The model under review builds one solid part; all positions refer to its coordinate system, in mm. Face numbers are marked on the shaded views. Round coordinates to 2 decimals unless told otherwise and drop trailing zeros. Loops run counter-clockwise (first coordinate to the right, second up) from the corner with the lowest first, then second, coordinate; pieces in that order, holes last. Notation, with made-up numbers: (-32, 39.5) -> (-9, 39.5) arc R5 cw to (-9, 48.5) -> close; hole circle Ø7 at (8, 71.25). An arc over 180 degrees is marked (long way). Return JSON: item names as keys, results as strings. Group by question number.
```python
from build123d import *

# Parameters (mm, degrees)
AUFSATZ_LINEAR_AUSTRAGEN1_DEPTH = 500


with BuildPart() as part:
    # Skizze1 → Aufsatz-Linear austragen1 (new body, symmetric)
    with BuildSketch(Plane(origin=(0, 0, 0), x_dir=(0, 0, -1), z_dir=(1, 0, 0))):
        with BuildLine():
            Line((-45.456738262, -1.013535579), (45.456738262, -1.013535579))
            Line((45.456738262, -1.013535579), (45.456738262, 7.828778751))
            ThreePointArc((45.456738262, 7.828778751), (44.798122061, 9.704391159), (43.111456992, 10.756464421))
            Line((43.111456992, 10.756464421), (22.36480763, 15.396040337))
            Line((22.36480763, 15.396040337), (9.658162352, 22.299803874))
            ThreePointArc((9.658162352, 22.299803874), (6.983652955, 24.872378626), (6, 28.45058603))
            Line((6, 28.45058603), (6, 85.036336881))
            ThreePointArc((6, 85.036336881), (9.227773203, 94.794679734), (17.637809302, 100.703577084))
            Line((17.637809302, 100.703577084), (32.825814996, 105.937662587))
            ThreePointArc((32.825814996, 105.937662587), (33.314191315, 106.302499454), (33.5, 106.883096132))
            Line((33.5, 106.883096132), (33.5, 124))
            ThreePointArc((33.5, 124), (29.399494937, 133.899494937), (19.5, 138))
            Line((19.5, 138), (-19.5, 138))
            ThreePointArc((-19.5, 138), (-29.399494937, 133.899494937), (-33.5, 124))
            Line((-33.5, 124), (-33.5, 106.883096132))
            ThreePointArc((-33.5, 106.883096132), (-33.314191315, 106.302499454), (-32.825814996, 105.937662587))
            Line((-32.825814996, 105.937662587), (-17.637809302, 100.703577084))
            ThreePointArc((-17.637809302, 100.703577084), (-9.227773203, 94.794679734), (-6, 85.036336881))
            Line((-6, 85.036336881), (-6, 28.45058603))
            ThreePointArc((-6, 28.45058603), (-6.983652955, 24.872378626), (-9.658162352, 22.299803874))
            Line((-9.658162352, 22.299803874), (-22.36480763, 15.396040337))
            Line((-22.36480763, 15.396040337), (-43.111456992, 10.756464421))
            ThreePointArc((-43.111456992, 10.756464421), (-44.798122061, 9.704391159), (-45.456738262, 7.828778751))
            Line((-45.456738262, 7.828778751), (-45.456738262, -1.013535579))
        make_face()
    extrude(amount=AUFSATZ_LINEAR_AUSTRAGEN1_DEPTH, both=True)


solid = part.part
```
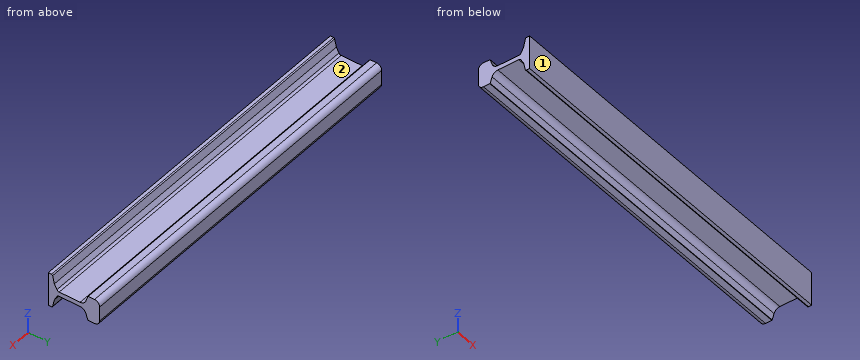
1. For P1, Ø5, axis at x = 114.5, y = 118.5, coming from the -Z side; P2, Ø1.5, axis at x = -59.5, z = 31.5, coming from the +Y side; P3, Ø6, axis at x = -250, z = 26.5, coming from the +Y side, all flat-tipped, find the tip position at first contact; note any pin that passes through.
2. We need section B-B, the plane y = 59. Write out the cut boundary in (x, z), then the cut area to 3 significant figures.
3. We need section A-A, the plane x = -301.5. Write out the cut boundary in (y, z), then the cut area to 3 significant figures.
4. Draft analysis for pull direction Y (two halves, no side actions). For the marked faces 1 and 2, state which applies: pulls with the +Y half, pulls with the -Y half, needs draft (parallel to the pull), parting line crosses it, or undercut.
5. Wall thickness on line 1 (Z direction, x = 222.5, y = 72); line 2 (Y direction, x = 66, z = 28.5); line 3 (Y direction, x = 449, z = -9): over which ranges is each line inside the solid? List them lowest first.
Check sheet entries:
{
 "1": {"P1": "stops at z = -33.5", "P2": "stops at y = 132.33", "P3": "stops at y = 137.42"},
 "2": {"outline": "(-500, -6) -> (500, -6) -> (500, 6) -> (-500, 6) -> close", "area": "12,000 mm²"},
 "3": {"outline": "(-1.01, -45.46) -> (7.83, -45.46) arc R3 ccw to (10.76, -43.11) -> (15.4, -22.36) -> (22.3, -9.66) arc R7 cw to (28.45, -6) -> (85.04, -6) arc R16.36 cw to (100.7, -17.64) -> (105.94, -32.83) arc R1 ccw to (106.88, -33.5) -> (124, -33.5) arc R14 ccw to (138, -19.5) -> (138, 19.5) arc R14 ccw to (124, 33.5) -> (106.88, 33.5) arc R1 ccw to (105.94, 32.83) -> (100.7, 17.64) arc R16.36 cw to (85.04, 6) -> (28.45, 6) arc R7 cw to (22.3, 9.66) -> (15.4, 22.36) -> (10.76, 43.11) arc R3 ccw to (7.83, 45.46) -> (-1.01, 45.46) -> close", "area": "4,970 mm²"},
 "4": {"face 1": "pulls with the -Y half", "face 2": "undercut"},
 "5": {"line 1": "z = -6 to 6", "line 2": "y = -1.01 to 14.02, 104.45 to 134.72", "line 3": "y = -1.01 to 22.71, 94.48 to 138"}
}
